```python
from build123d import *

# Parameters (mm, degrees)
ESQUISSE1_W                     = 48
ESQUISSE1_H                     = 63.5
BOSS_EXTRU_1_DEPTH              = 4
CONG_1_R                        = 1
DIAM_TRE_DU_PER_AGE_22_0_22_1_D = 22
D_GAGEMENT_M31_D                = 3.6
R_P_TITION_LIN_AIRE1_COUNT      = 2
R_P_TITION_LIN_AIRE1_PITCH      = 31
R_P_TITION_LIN_AIRE2_COUNT      = 2
R_P_TITION_LIN_AIRE2_PITCH      = 31
R_P_TITION_LIN_AIRE2_COPY_1_D   = 3.6
D_GAGEMENT_M2_54_D              = 3.1
ESQUISSE19_W                    = 18.410058986
ESQUISSE19_H                    = 2.5
ESQUISSE19_W_2                  = 24.589941014
BOSS_EXTRU_2_DEPTH              = 15
CONG_2_R                        = 5


with BuildPart() as part:
    # Esquisse1 → Boss.-Extru.1 (new body)
    with BuildSketch(Plane.XY):
        with Locations((9.64559387, 37.224137931)):
            Rectangle(ESQUISSE1_W, ESQUISSE1_H)
    extrude(amount=BOSS_EXTRU_1_DEPTH)

    # Congé1
    cong_1_edges = [part.edges().sort_by_distance(p)[0] for p in [
        (9.64559387, 68.974137931, 0),
        (33.64559387, 37.224137931, 0),
        (9.64559387, 5.474137931, 0),
        (-14.35440613, 37.224137931, 0),
    ]]
    fillet(cong_1_edges, radius=CONG_1_R)

    # Diamètre du perçage Ø22.0 (22)1 (through all)
    with Locations(Plane.XY.offset(4)):
        with Locations((9.64559387, 29.474137931)):
            Hole(DIAM_TRE_DU_PER_AGE_22_0_22_1_D / 2)

    # Dégagement M31 (through all)
    with Locations(Plane.XY.offset(4)):
        with Locations((-5.85440613, 44.974137931)):
            d_gagement_m31 = Hole(D_GAGEMENT_M31_D / 2)

    # Répétition linéaire1: Dégagement M31 ×2
    with Locations(*[(i * R_P_TITION_LIN_AIRE1_PITCH, 0, 0) for i in range(1, R_P_TITION_LIN_AIRE1_COUNT)]):
        add(d_gagement_m31, mode=Mode.SUBTRACT)

    # Répétition linéaire2: Dégagement M31 ×2
    with Locations(*[(0, -i * R_P_TITION_LIN_AIRE2_PITCH, 0) for i in range(1, R_P_TITION_LIN_AIRE2_COUNT)]):
        add(d_gagement_m31, mode=Mode.SUBTRACT)

    # Répétition linéaire2 copy 1 (through all)
    with Locations(Plane(origin=(31, -31, 4), x_dir=(1, 0, 0), z_dir=(0, 0, 1))):
        with Locations((-5.85440613, 44.974137931)):
            Hole(R_P_TITION_LIN_AIRE2_COPY_1_D / 2)

    # Dégagement M2.54 (through all)
    with Locations(Plane.XY.offset(4)):
        with Locations((-4.35440613, 60.474137931), (23.64559387, 60.474137931)):
            Hole(D_GAGEMENT_M2_54_D / 2)

    # Esquisse19 → Boss.-Extru.2 (add)
    with BuildSketch(Plane.XY.offset(4)):
        Polygon((-14.35440613, 50.474137931), (-14.35440613, 5.474137931), (-11.85440613, 5.474137931), (-11.85440613, 7.974137931), (-11.85440613, 50.474137931), align=None)
        with Locations((-2.649376637, 6.724137931)):
            Rectangle(ESQUISSE19_W, ESQUISSE19_H)
        with Locations((18.850623363, 6.724137931)):
            Rectangle(ESQUISSE19_W_2, ESQUISSE19_H)
        Polygon((31.14559387, 7.974137931), (31.14559387, 5.474137931), (33.64559387, 5.474137931), (33.64559387, 50.474137931), (31.14559387, 50.474137931), align=None)
    extrude(amount=BOSS_EXTRU_2_DEPTH)

    # Congé2
    # the kernel refuses this fillet: 5 mm, written as the material it takes off along each edge
    with BuildSketch(Plane(origin=(-9.35440613, 10.474137931, 0), x_dir=(0, -1, 0), z_dir=(1, 0, 0))) as cong_2_piece_1:
        with BuildLine():
            CenterArc((4, -1), 1, 0, 90)
            Line((5, -1), (5, 0))
            Line((5, 0), (4, 0))
        make_face()
    revolve(axis=Axis((-9.35440613, 10.474137931, 0), (0, 0, -1)), revolution_arc=90, mode=Mode.SUBTRACT)
    with BuildSketch(Plane(origin=(28.64559387, 10.474137931, 0), x_dir=(1, 0, 0), z_dir=(0, 1, 0))) as cong_2_piece_2:
        with BuildLine():
            CenterArc((4, -1), 1, 0, 90)
            Line((5, -1), (5, 0))
            Line((5, 0), (4, 0))
        make_face()
    revolve(axis=Axis((28.64559387, 10.474137931, 0), (0, 0, -1)), revolution_arc=90, mode=Mode.SUBTRACT)
    with BuildSketch(Plane(origin=(33.64559387, 5.474137931, 31.5), x_dir=(0, 1, 0), z_dir=(0, 0, -1))) as cong_2_piece_3:
        with BuildLine():
            CenterArc((CONG_2_R, -CONG_2_R), CONG_2_R, 90, 90)
            Line((0, -CONG_2_R), (0, 0))
            Line((0, 0), (CONG_2_R, 0))
        make_face()
    extrude(amount=31.5, mode=Mode.SUBTRACT)
    with BuildSketch(Plane(origin=(-14.35440613, 5.474137931, 0), x_dir=(1, 0, 0), z_dir=(0, 0, 1))) as cong_2_piece_4:
        with BuildLine():
            CenterArc((CONG_2_R, CONG_2_R), CONG_2_R, 180, 90)
            Line((0, CONG_2_R), (0, 0))
            Line((0, 0), (CONG_2_R, 0))
        make_face()
    extrude(amount=31.5, mode=Mode.SUBTRACT)


solid = part.part
```
Input: part model. Units: mm. Frame: model coordinates. A direction names the side the tool comes from. Round coordinates to 2 decimals unless told otherwise and drop trailing zeros. Write each loop counter-clockwise with the first axis right and the second up, starting at its lowest first coordinate (ties: lowest second). Pieces come first, ordered by that corner, then holes. Notation, with made-up numbers: (66.25, 10.5) -> (114.25, 10.5) arc R19 ccw to (114.25, 17.5) -> close; hole circle Ø6 at (83, -6). An arc over 180 degrees is marked (long way). Answer as CSV lines item,"result".
1. Section A-A (x = 3.5). Return the cut outline in (y, z).
Geometry says:
outline,"(5.47, 1) arc R1 ccw to (6.47, 0) -> (20.35, 0) -> (20.35, 4) -> (7.97, 4) -> (7.97, 19) -> (5.47, 19) -> close; (38.6, 0) -> (67.97, 0) arc R1 ccw to (68.97, 1) -> (68.97, 4) -> (38.6, 4) -> close"
2. Section C-C (z = 3). Return the cut outline in (x, y), plus the area to 3 significant figures.
Geometry says:
outline,"(-14.35, 10.47) arc R5 ccw to (-9.35, 5.47) -> (28.65, 5.47) arc R5 ccw to (33.65, 10.47) -> (33.65, 68.97) -> (-14.35, 68.97) -> close; hole circle Ø3.6 at (-5.85, 13.97); hole circle Ø3.6 at (-5.85, 44.97); hole circle Ø3.1 at (-4.35, 60.47); hole circle Ø22 at (9.65, 29.47); hole circle Ø3.1 at (23.65, 60.47); hole circle Ø3.6 at (25.15, 13.97); hole circle Ø3.6 at (25.15, 44.97)"
area,"2,600 mm^2"
3. Contact query for flat-ended pins moving along their axis: P1, Ø4, axis at x = -5.85, y = 44.97, coming from the +Z side; P2, Ø8, axis at x = 3.5, z = 15.5, coming from the +Y side; P3, Ø3, axis at x = 32.5, z = 12, coming from the +Y side. Output: stop coordinate, or through.
Geometry says:
P1,"stops at z = 4"
P2,"stops at y = 7.97"
P3,"stops at y = 50.47"
4. Ray query, L1, parallel to X at y = 47, z = 14.25; L2, parallel to Y at x = -4, z = 13.5; L3, parallel to X at y = 30, z = 1.75. Return the intervals inside material, ascending. Write a range as [from, to].
Geometry says:
L1,"x = [-14.35, -11.85], [31.15, 33.65]"
L2,"y = [5.47, 7.97]"
L3,"x = [-14.35, -1.34], [20.63, 33.65]"
5. Reachability of faces 5 (the cylindrical face through (-5.62, 15.76, 1.97)), 6 (the flat face through (31.146, 30, 11)), 7 (the flat face through (32, 50.474, 11)) from +Z, -Z, +X, -X, +Y, -Y: full face, straight path, thin tool, end or side. Return the list, or none.
Geometry says:
face 5,"+Z, -Z"
face 6,"+Z, +Y"
face 7,"+Z, +X, -X, +Y"
6. Section B-B (y = 17). Return the cut outline in (x, z).
Geometry says:
outline,"(-14.35, 1) arc R1 ccw to (-13.35, 0) -> (32.65, 0) arc R1 ccw to (33.65, 1) -> (33.65, 19) -> (31.15, 19) -> (31.15, 4) -> (-11.85, 4) -> (-11.85, 19) -> (-14.35, 19) -> close"
7. Mould query, pull axis Y, two halves, no side actions, for faces 1 (the flat face through (-13, 50.474, 11)), 2 (the flat face through (10, 6, 19)), 3 (the cylindrical face through (22.167, 60.94, 1.972)), 4 (the cylindrical face through (26.944, 45.053, 1.972)). Classes: +Y half, -Y half, draft (parallel to the pull), parting line (faces both ways), or undercut.
Geometry says:
face 1,"+Y half"
face 2,"draft"
face 3,"undercut"
face 4,"undercut"
8. Section D-D (z = 11). Return the cut outline in (x, y), plus the area to 3 significant figures.
Geometry says:
outline,"(-14.35, 10.47) arc R5 ccw to (-9.35, 5.47) -> (28.65, 5.47) arc R5 ccw to (33.65, 10.47) -> (33.65, 50.47) -> (31.15, 50.47) -> (31.15, 7.97) -> (-11.85, 7.97) -> (-11.85, 50.47) -> (-14.35, 50.47) -> close"
area,"322 mm^2"
